The listing builds one solid part. Answer for the finished solid, in the listing's coordinates (mm). Face numbers are marked on the shaded views. Round coordinates to 2 decimals unless told otherwise and drop trailing zeros. Write each loop counter-clockwise with the first axis right and the second up, starting at its lowest first coordinate (ties: lowest second). Pieces come first, ordered by that corner, then holes.
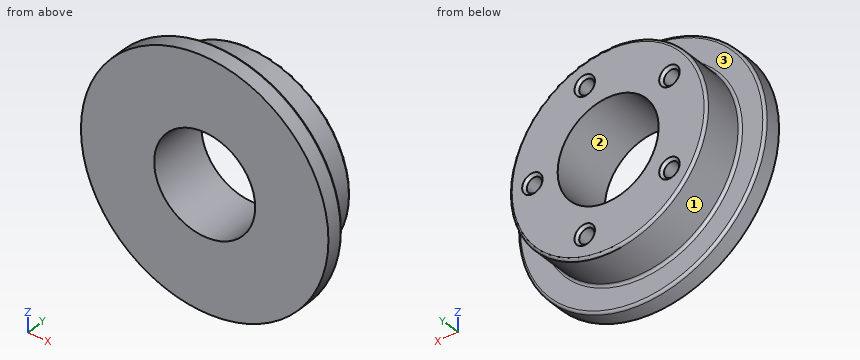
from build123d import *

# Parameters (mm, degrees)
SKETCH1_R          = 24.5
SKETCH1_R_2        = 10
EXTRUDE1_DEPTH     = 3.5
SKETCH1_3_R        = 19.5
SKETCH1_3_R_2      = 10
EXTRUDE2_DEPTH     = 12
CIRPATTERN1_COUNT  = 5
FINISHING_FILLET_R = 0.5


with BuildPart() as part:
    # Sketch1 → Extrude1 (new body)
    with BuildSketch(Plane(origin=(0, 0, 0), x_dir=(1, 0, 0), z_dir=(0, 1, 0))):
        Circle(SKETCH1_R)
        Circle(SKETCH1_R_2, mode=Mode.SUBTRACT)
    extrude(amount=EXTRUDE1_DEPTH)

    # Sketch1_3 → Extrude2 (add)
    with BuildSketch(Plane(origin=(0, 0, 0), x_dir=(1, 0, 0), z_dir=(0, 1, 0))):
        Circle(SKETCH1_3_R)
        Circle(SKETCH1_3_R_2, mode=Mode.SUBTRACT)
    extrude(amount=EXTRUDE2_DEPTH)

    # Sketch3 → 3.0 Diameter Hole1 (revolve, cut)
    with BuildSketch(Plane(origin=(15, 12, 0), x_dir=(0, 0, 1), z_dir=(1, 0, 0))):
        Polygon((0, 0), (0, 10.901290929), (1.5, 10), (1.5, 0.525), (2.025, 0), align=None)
    f_3_0_diameter_hole1 = revolve(axis=Axis((15, 18.35, 0), (0, -1, 0)), mode=Mode.SUBTRACT)

    # CirPattern1: 3.0 Diameter Hole1 ×5 about axis
    cirpattern1_axis = Axis((0, 0, 0), (0, 1, 0))
    for i in range(1, CIRPATTERN1_COUNT):
        add(f_3_0_diameter_hole1.rotate(cirpattern1_axis, i * 360 / CIRPATTERN1_COUNT), mode=Mode.SUBTRACT)

    # Finishing Fillet
    finishing_fillet_edges = [part.edges().sort_by_distance(p)[0] for p in [
        (-19.5, 3.5, 0),
        (-19.5, 12, 0),
        (-24.5, 3.5, 0),
    ]]
    fillet(finishing_fillet_edges, radius=FINISHING_FILLET_R)


solid = part.part
1. For a pull along Z with two mould halves and no side action, classify the marked faces 1, 2 and 3 as released by +Z, released by -Z, zero draft, split by the parting line, or undercut.
Geometry says:
face 1: split by the parting line
face 2: undercut
face 3: zero draft
2. Straight lines are drawn through the part: line 1 along X through (y, z) = (9.5, 1); line 2 along Z through (x, y) = (-13, 7.25); line 3 along Z through (x, y) = (0, 7.75). For each, find the intervals that lie inside material, in ascending order.
Geometry says:
line 1: x = -19.47 to -9.95, 9.95 to 13.88, 16.12 to 19.47
line 2: z = -14.53 to -10.04, -7.59 to 7.59, 10.04 to 14.53
line 3: z = -19.5 to -10, 10 to 19.5
3. Given pin 1 (3 mm diameter, centred on x = -14.5, y = 4.5, fed in from +Z); pin 2 (6 mm diameter, centred on x = -3.5, y = 5, fed in from +Z); pin 3 (1.5 mm diameter, centred on x = 12, y = 9.5, fed in from -Z), each flat-ended and moving along its own axis, determine where each tip first touches the part or whether it passes through.
Geometry says:
pin 1: stops at z = 20.26
pin 2: stops at z = 24.47
pin 3: stops at z = -15.93
4. Section A-A on x = 0 is taken. Determine the outline of the cut face in (y, z), plus the area to 3 significant figures.
Geometry says:
outline: (0, -24.5) - (3, -24.5) arc R0.5 ccw to (3.5, -24) - (3.5, -20) arc R0.5 cw to (4, -19.5) - (11.5, -19.5) arc R0.5 ccw to (12, -19) - (12, -10) - (0, -10) - close; (0, 10) - (12, 10) - (12, 19) arc R0.5 ccw to (11.5, 19.5) - (4, 19.5) arc R0.5 cw to (3.5, 20) - (3.5, 24) arc R0.5 ccw to (3, 24.5) - (0, 24.5) - close
area: 263 mm2
5. Section B-B on y = 5.75 is taken. Determine the outline of the cut face in (x, z).
Geometry says:
outline: circle Ø39 at (0, 0); hole circle Ø3 at (-12.14, -8.82); hole circle Ø3 at (-12.14, 8.82); hole circle Ø20 at (0, 0); hole circle Ø3 at (4.64, -14.27); hole circle Ø3 at (4.64, 14.27); hole circle Ø3 at (15, 0)
